Source: CAD feature listing. Evaluate the final solid. Frame: model axes, mm. A direction names the side the tool comes from. Give positions to 0.01 mm unless a question says otherwise; leave off trailing zeros. Order: outer loops, then holes, each group sorted by start corner. A loop starts at its lowest first (then second) coordinate and runs counter-clockwise, first axis right, second up.
from build123d import *

# Parameters (mm, degrees)
SKETCH2_R           = 10.5
SKETCH2_R_2         = 8
BOSS_EXTRUDE1_DEPTH = 114
BOSS_EXTRUDE2_START = 36
SKETCH4_R           = 9
SKETCH4_R_2         = 8
BOSS_EXTRUDE2_DEPTH = 36


with BuildPart() as part:
    # Sketch2 → Boss-Extrude1 (new body)
    with BuildSketch(Plane.XY):
        with Locations(Location((0, 0, 0), (0, 0, 180))):
            Circle(SKETCH2_R)
        with Locations(Location((0, 0, 0), (0, 0, 180))):
            Circle(SKETCH2_R_2, mode=Mode.SUBTRACT)
    extrude(amount=BOSS_EXTRUDE1_DEPTH)

    # Sketch4 → Boss-Extrude2 (add)
    with BuildSketch(Plane(origin=(0, 0, 0), x_dir=(-1, 0, 0), z_dir=(0, 0, -1)).offset(BOSS_EXTRUDE2_START)):
        Circle(SKETCH4_R)
        Circle(SKETCH4_R_2, mode=Mode.SUBTRACT)
    extrude(amount=-BOSS_EXTRUDE2_DEPTH)


solid = part.part
1) Section query D-D on z = -22.5. Output: boundary loops of the cut face in (x, y).
Checks:
outline: circle Ø18 at (0, 0); hole circle Ø16 at (0, 0)
2) First-contact query: pin 1 Ø8 at (y, z) = (-7.5, 79) entering from -X; pin 2 Ø10 at (x, y) = (-0.5, 6) entering from -Z; pin 3 Ø8 at (x, z) = (4, -2) entering from -Y; pin 4 Ø12 at (y, z) = (8.5, 46) entering from -X. Flat tips, straight axial feed; report the tip coordinate or a pass-through.
Checks:
pin 1: stops at x = -9.9
pin 2: stops at z = -36
pin 3: stops at y = -10.49
pin 4: stops at x = -10.2
3) Reachability of faces 1 (the face through (2, 8, 114)), 2 (the face through (-8, -5, 0)) from +Z, -Z, +X, -X, +Y, -Y: full face, straight path, thin tool, end or side. Return the list, or none.
Checks:
face 1: +Z, +X, -X, +Y, -Y
face 2: -Z
4) Ray query, L1, parallel to Y at x = 0, z = 85; L2, parallel to Y at x = 0, z = -16; L3, parallel to Z at x = -7, y = -7. Return the intervals inside material, ascending.
Checks:
L1: y = -10.5 to -8, 8 to 10.5
L2: y = -9 to -8, 8 to 9
L3: z = 0 to 114
5) Section query C-C on z = 63. Output: boundary loops of the cut face in (x, y).
Checks:
outline: circle Ø21 at (0, 0); hole circle Ø16 at (0, 0)
6) Section query A-A on x = 0. Output: boundary loops of the cut face in (y, z).
Checks:
outline: (-10.5, 0) - (-9, 0) - (-9, -36) - (-8, -36) - (-8, 114) - (-10.5, 114) - close; (8, -36) - (9, -36) - (9, 0) - (10.5, 0) - (10.5, 114) - (8, 114) - close
